Part model, mm, in its own coordinate system. Face numbers are marked on the shaded views. Coordinates: 2 decimals unless noted, no trailing zeros. Write each loop counter-clockwise with the first axis right and the second up, starting at its lowest first coordinate (ties: lowest second). Pieces come first, ordered by that corner, then holes. Notation, with made-up numbers: (-18.5, -31.75) - (40.5, -31.75) arc R21 ccw to (40.5, -15.75) - close; hole circle Ø1 at (37, 34.5). An arc over 180 degrees is marked (long way). Use a Markdown table: item, result.
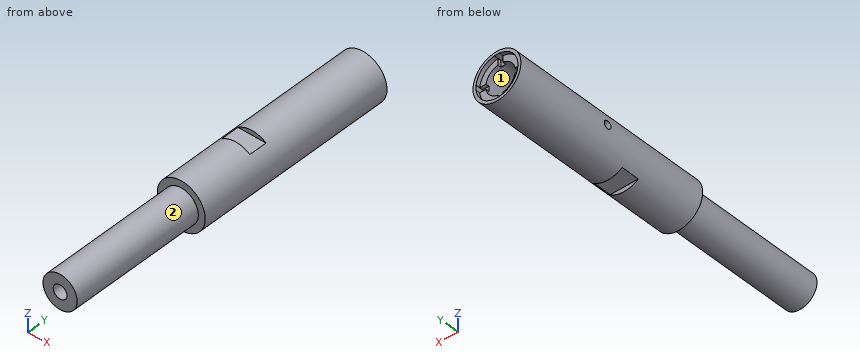
```python
from build123d import *

# Parameters (mm, degrees)
F0_R      = 10.5
F1_DEPTH  = 90
F2_R      = 7.5
F3_DEPTH  = 60
F5_D      = 6
F6_R      = 4.75
F6_R_2    = 3
F7_DEPTH  = 50
F8_R      = 6.45
F9_DEPTH  = 21
F10_R     = 9.2
F11_DEPTH = 1.75
F12_W     = 8.1
F12_H     = 2.2
F13_DEPTH = 3.25
F15_W     = 49.0491833104
F15_H     = 8
F16_DEPTH = 2
F18_W     = 39.7552206603
F18_H     = 8
F19_DEPTH = 2
F22_D     = 3.3
F22_DEPTH = 10
F22_TIP   = 0.9914200214


with BuildPart() as f1:
    # F0 (on Front) → F1 (new body)
    with BuildSketch(Plane.XZ):
        Circle(F0_R)
    extrude(amount=F1_DEPTH)

    # F2 (on face) → F3 (join)
    with BuildSketch(Plane.XZ.offset(90)):
        Circle(F2_R)
    extrude(amount=F3_DEPTH)

    # F5 (through all)
    with Locations(Plane.XZ.offset(150)):
        with Locations((0, 0)):
            Hole(F5_D / 2)

    # F6 (on face) → F7 (cut)
    with BuildSketch(Plane(origin=(0, 0, 0), x_dir=(-1, 0, 0), z_dir=(0, 1, 0))):
        Circle(F6_R)
        Circle(F6_R_2, mode=Mode.SUBTRACT)
    extrude(amount=-F7_DEPTH, mode=Mode.SUBTRACT)

    # F8 (on face) → F9 (cut)
    with BuildSketch(Plane(origin=(0, 0, 0), x_dir=(-1, 0, 0), z_dir=(0, 1, 0))):
        Circle(F8_R)
    extrude(amount=-F9_DEPTH, mode=Mode.SUBTRACT)

    # F10 (on Front) → F11 (cut)
    with BuildSketch(Plane.XZ):
        Circle(F10_R)
    extrude(amount=F11_DEPTH, mode=Mode.SUBTRACT)

    # F12 (on Front) → F13 (cut)
    with BuildSketch(Plane.XZ):
        Polygon((1.0996337654, -1.1), (1.0996337654, 0), (1.0996337654, 1.1), (0, 1.1), (-1.1, 1.1), (-1.1, -1.1), (0, -1.1), align=None)
        Polygon((1.0996337654, 1.1), (1.0996337654, 0), (1.0996337654, -1.1), (9.2, -1.1), (9.2, 1.1), align=None)
        Polygon((0, 1.1), (1.0996337654, 1.1), (1.0996337654, 9.2), (-1.1, 9.2), (-1.1, 1.1), align=None)
        Polygon((1.0996337654, -9.2), (1.0996337654, -1.1), (0, -1.1), (-1.1, -1.1), (-1.1, -9.2), align=None)
        with Locations((-5.15, 0)):
            Rectangle(F12_W, F12_H)
    extrude(amount=F13_DEPTH, mode=Mode.SUBTRACT)

    # F15 (on offset) → F16 (cut)
    with BuildSketch(Plane.XY.offset(10.5)):
        with Locations((-2.6939958334, -59)):
            Rectangle(F15_W, F15_H)
    extrude(amount=-F16_DEPTH, mode=Mode.SUBTRACT)

    # F18 (on offset) → F19 (cut)
    with BuildSketch(Plane.XY.offset(-10.5)):
        with Locations((0.5775718018, -59)):
            Rectangle(F18_W, F18_H)
    extrude(amount=F19_DEPTH, mode=Mode.SUBTRACT)

    # F22
    with Locations(Plane(origin=(-10.5, 0, 0), x_dir=(0, 1, 0), z_dir=(-1, 0, 0))):
        with Locations((-43, 0)):
            Hole(F22_D / 2, depth=F22_DEPTH)
            with Locations((0, 0, -(F22_DEPTH + F22_TIP / 2))):  # 118° drill point
                Cone(0, F22_D / 2, F22_TIP, mode=Mode.SUBTRACT)


solid = f1.part
```
Item 1: Drill centre lines: probe 1 along Y at (x, z) = (-5.25, -8.75); probe 2 along X at (y, z) = (-7, 0); probe 3 along Z at (x, y) = (0, -36). Where is each one in solid material? Low to high.
From the geometry:
| item | result |
|---|---|
| probe 1 | -90 to -63, -55 to 0 |
| probe 2 | -10.5 to -6.45, 6.45 to 10.5 |
| probe 3 | -10.5 to -4.75, 4.75 to 10.5 |
Item 2: Drop flat-ended pins along their axis: P1, Ø1.4, axis at y = -2, z = -7.5, coming from the -X side; P2, Ø5, axis at x = 1, z = -0.5, coming from the +Y side; P3, Ø8, axis at y = -111, z = -6, coming from the -X side. Give the stop position or say it passes through.
From the geometry:
| item | result |
|---|---|
| P1 | x = -8 |
| P2 | y = -50 |
| P3 | x = -7.23 |
Item 3: Two-plate mould, pull along X, no slides. Class the marked faces 1 and 2: pulls with the +X half, pulls with the -X half, needs draft (parallel to the pull), parting line crosses it, or undercut.
From the geometry:
| item | result |
|---|---|
| face 1 | undercut |
| face 2 | parting line crosses it |
Item 4: Band-saw the part on A-A, the plane y = -36.5. Give the cut face in (x, z), then the cut area to 3 significant figures.
From the geometry:
| item | result |
|---|---|
| outline | circle Ø21 at (0, 0); hole circle Ø9.5 at (0, 0) |
| area | 275 mm^2 |
